```python
from build123d import *

# Parameters (mm, degrees)
F0_R     = 25.4
F1_DEPTH = 190.5
F3_DEPTH = 19.05
F5_DEPTH = 19.05
F6_R     = 2.54
F7_R     = 2.54
F8_R     = 1.27
F9_R     = 1.27


with BuildPart() as f1:
    # F0 (on Right) → F1 (new body)
    with BuildSketch(Plane.YZ):
        Circle(F0_R)
    extrude(amount=F1_DEPTH)

    # F2 (on face) → F3 (join)
    with BuildSketch(Plane(origin=(0, 0, 0), x_dir=(0, -1, 0), z_dir=(-1, 0, 0))):
        Polygon((5.499261, 9.525), (-5.499261, 9.525), (-10.998523, 0), (-5.499261, -9.525), (5.499261, -9.525), (10.998523, 0), align=None)
    extrude(amount=F3_DEPTH)

    # F4 (on face) → F5 (join)
    with BuildSketch(Plane.YZ.offset(190.5)):
        Polygon((10.998121, -0.093942), (5.580416, 9.477682), (-5.417705, 9.571623), (-10.998121, 0.093942), (-5.580416, -9.477682), (5.417705, -9.571623), align=None)
    extrude(amount=F5_DEPTH)

    # F6
    f6_edges = [f1.edges().sort_by_distance(p)[0] for p in [
        (190.5, -25.4, 0),
    ]]
    fillet(f6_edges, radius=F6_R)

    # F7
    f7_edges = [f1.edges().sort_by_distance(p)[0] for p in [
        (0, -25.4, 0),
    ]]
    fillet(f7_edges, radius=F7_R)

    # F8
    f8_edges = [f1.edges().sort_by_distance(p)[0] for p in [
        (209.55, 8.289269, 4.69187),
        (209.55, 0.081356, 9.524653),
        (209.55, -8.207913, 4.832782),
        (209.55, -8.289269, -4.69187),
        (209.55, -0.081356, -9.524653),
        (209.55, 8.207913, -4.832782),
    ]]
    fillet(f8_edges, radius=F8_R)

    # F9
    f9_edges = [f1.edges().sort_by_distance(p)[0] for p in [
        (-19.05, 0, 9.525),
        (-19.05, 8.248892, 4.7625),
        (-19.05, 8.248892, -4.7625),
        (-19.05, 0, -9.525),
        (-19.05, -8.248892, -4.7625),
        (-19.05, -8.248892, 4.7625),
    ]]
    fillet(f9_edges, radius=F9_R)


solid = f1.part
```
Input: part model. Units: mm. Frame: model coordinates. A direction names the side the tool comes from. Round coordinates to 2 decimals unless told otherwise and drop trailing zeros. Order: outer loops, then holes, each group sorted by start corner. A loop starts at its lowest first (then second) coordinate and runs counter-clockwise, first axis right, second up. Notation, with made-up numbers: (35, -1) - (75, -1) arc R24 ccw to (75, 35) - close; hole circle Ø4 at (-10.75, -3). An arc over 180 degrees is marked (long way). One line per question, with ' | ' between items. Start each with the question number.
1) Contact query for flat-ended pins moving along their axis: P1, Ø4, axis at x = 79.5, y = 9, coming from the +Z side; P2, Ø10, axis at y = -2, z = -19.5, coming from the +X side; P3, Ø12, axis at x = -10.5, y = 2, coming from the +Z side (3 decimals). Output: stop coordinate, or through.
2) Cut plane A-A, the plane x = 125. Return the cut outline in (y, z).
3) Ray query, probe 1 along X at (y, z) = (4.5, -22.5); probe 2 along Y at (x, z) = (135, 0.5); probe 3 along X at (y, z) = (7, 4.5). Return the intervals inside material, ascending.
4) Set-up query: faces 1 (the flat face through (-9, 0, 9.525)), 2 (the flat face through (199.27, -8.17, 4.9)), 3 (the flat face through (-9, 0, -9.525)). Return all of +Z, -Z, +X, -X, +Y, -Y with unobstructed straight access to the full face (end or side cutting, diameter ignored); none if empty.
Worked out:
1) P1: stops at z = 24.42 | P2: stops at x = 190.5 | P3: stops at z = 9.525
2) outline: circle Ø50.8 at (0, 0)
3) probe 1: x = 0 to 190.5 | probe 2: y = -25.4 to 25.4 | probe 3: x = -19.05 to 209.55
4) face 1: +Z, -X, +Y, -Y | face 2: +Z, +X, -Y | face 3: -Z, -X, +Y, -Y
